Autodesk Inventor part; units mm, degrees
ref_plane "YZ Plane" through (0, 0, 0) normal (1, 0, 0) x (0, 1, 0)
ref_plane "XZ Plane" through (0, 0, 0) normal (0, 1, 0) x (-1, 0, 0)
ref_plane "XY Plane" through (0, 0, 0) normal (0, 0, 1) x (1, 0, 0)
sketch "Sketch1" plane through (0, 0, 0) normal (0, 1, 0) x (-1, 0, 0)
  line L0 (107.2514, 61.1758) -> (-112.4586, 61.1758)
  line L1 (-112.4586, 61.1758) -> (-112.4586, 42.1258)
  line L2 (-112.4586, 42.1258) -> (107.2514, 42.1258)
  line L3 (107.2514, 42.1258) -> (107.2514, 61.1758)
  point P0 (0, 0)
  dimension "d0" = 219.71
  dimension "d1" = 19.05
extrude "Extrusion1" add sketch "Sketch1" along normal blind 50.8
sketch "Sketch2" plane through (-107.2514, 0, 61.1758) normal (0, 0, 1) x (1, 0, 0)
  line L0 (0, 0) -> (219.71, 0)
  line L1 (0, 50.8) -> (219.71, 50.8)
  line L2 (0, 0) -> (0, 50.8)
  line L3 (219.71, 0) -> (219.71, 50.8)
  point P0 (107.2514, 0)
  point P1 (9.525, 38.1)
  point P2 (9.525, 12.7)
  point P3 (210.185, 12.7)
  point P4 (210.185, 38.1)
  dimension "d4" = 0
  dimension "d5" = 0
  dimension "d6" = 0
  dimension "d7" = 0
  dimension "d8" = 12.7
  dimension "d9" = 12.7
  dimension "d10" = 9.525
  dimension "d11" = 9.525
hole "Hole1" at (-97.7264, 38.1, 61.1758) at (-97.7264, 12.7, 61.1758) at (102.9336, 12.7, 61.1758) at (102.9336, 38.1, 61.1758) direction (0, 0, -1) diameter 6.35 end through all
sketch "Sketch3" plane through (-107.2514, 0, 61.1758) normal (0, 0, 1) x (1, 0, 0)
  line L0 (19.05, 44.45) -> (200.66, 44.45)
  line L1 (200.66, 44.45) -> (200.66, 6.35)
  line L2 (200.66, 6.35) -> (19.05, 6.35)
  line L3 (19.05, 6.35) -> (19.05, 44.45)
  line L4 (0, 0) -> (0, 50.8)
  line L5 (219.71, 0) -> (219.71, 50.8)
  line L6 (219.71, 50.8) -> (0, 50.8)
  line L7 (0, 0) -> (219.71, 0)
  point P0 (107.2514, 0)
  dimension "d19" = 19.05
  dimension "d20" = 19.05
  dimension "d21" = 6.35
  dimension "d22" = 6.35
extrude "Extrusion2" cut sketch "Sketch3" against normal blind 6.35 contours L0 L1 L2 L3
sketch "Sketch6" plane through (0, 50.8, 0) normal (0, 1, 0) x (1, 0, 0)
  line L0 (-88.2014, -54.8258) -> (-107.2514, -54.8258)
  line L1 (-107.2514, -54.8258) -> (-107.2514, -42.1258)
  line L2 (-107.2514, -42.1258) -> (-88.2014, -42.1258)
  line L3 (-88.2014, -42.1258) -> (-88.2014, -54.8258)
  line L4 (112.4586, -42.1258) -> (-107.2514, -42.1258)
  line L5 (-107.2514, -42.1258) -> (-107.2514, -61.1758)
  line L6 (112.4586, -54.8258) -> (93.4086, -54.8258)
  line L7 (93.4086, -54.8258) -> (93.4086, -42.1258)
  line L8 (93.4086, -42.1258) -> (112.4586, -42.1258)
  line L9 (112.4586, -42.1258) -> (112.4586, -54.8258)
  line L10 (112.4586, -61.1758) -> (112.4586, -42.1258)
  line L11 (-107.2514, -61.1758) -> (112.4586, -61.1758)
  point P0 (0, 0)
  dimension "d25" = 0
  dimension "d26" = 12.7
  dimension "d27" = 0
  dimension "d28" = 19.05
  dimension "d32" = 19.05
  dimension "d33" = 0
  dimension "d34" = 6.35
extrude "Extrusion3" cut sketch "Sketch6" against normal blind 76.2 contours L0 L1 L2 L3 | L4 L9 L6 L7
sketch "Sketch7" plane through (0, 0, 0) normal (0, -1, 0) x (1, 0, 0)
  line L0 (112.4586, 61.1758) -> (112.4586, 54.8258)
  line L1 (93.4086, 42.1258) -> (-88.2014, 42.1258)
  line L2 (-107.2514, 54.8258) -> (-107.2514, 61.1758)
  point P0 (0, 0)
  point P1 (61.6586, 51.6508)
  point P2 (-56.4514, 51.6508)
  dimension "d37" = 50.8
  dimension "d38" = 9.525
  dimension "d39" = 50.8
  dimension "d40" = 9.525
hole "Hole2" at (61.6586, 0, 51.6508) at (-56.4514, 0, 51.6508) direction (0, 1, 0) diameter 4.9149 depth 25.4 tip angle 118
sketch "Sketch8" plane through (0, 0, 0) normal (0, -1, 0) x (1, 0, 0)
  line L0 (112.4586, 61.1758) -> (112.4586, 54.8258)
  line L1 (93.4086, 42.1258) -> (-88.2014, 42.1258)
  point P0 (0, 0)
  point P1 (-1.8414, 51.6508)
  point P2 (-1.8414, 51.6508)
  dimension "d48" = 114.3
  dimension "d49" = 9.525
hole "Hole3" at (-1.8414, 0, 51.6508) direction (0, 1, 0) diameter 4.9149 depth 25.4 tip angle 118
properties part number "BottomWall"
Can you work these out from the model? Positions are in its coordinate system, mm. A direction names the side the tool comes from. Give positions to 0.01 mm unless a question says otherwise; leave off trailing zeros. Order: outer loops, then holes, each group sorted by start corner. A loop starts at its lowest first (then second) coordinate and runs counter-clockwise, first axis right, second up. Notation, with made-up numbers: (47.25, 87.5) - (53.25, 87.5) arc R10 ccw to (53.25, 106.5) - close; hole circle Ø1 at (56, -16). An arc over 180 degrees is marked (long way). Write each question's results on one line, items separated by ' | '.
1) On a 3-axis mill with a long thin cutter (end or side, diameter ignored), from which of +Z, -Z, +X, -X, +Y, -Y can I reach the whole of each face in a straight line? I mean faces 4 (the face through (-88.201, 25, 58)), 5 (the face through (-2.58, 12.878, 49.307)), 6 (the face through (-100.874, 13.113, 57.956)), 7 (the face through (-98, 26, 54.826)), 8 (the face through (93.409, 26, 49)). Say none if no direction works.
Final values:
face 4: +Z | face 5: -Y | face 6: +Z, -Z | face 7: -Z, -X, +Y, -Y | face 8: -Z, +X, +Y, -Y
2) Please list where these lines run through material, in increasing order: line 1 along X through (y, z) = (9, 52); line 2 along X through (y, z) = (38.1, 57.5); line 3 along Y through (x, z) = (-60.5, 60). Write a range as [from, to].
Final values:
line 1: x = [-88.2, -58.88], [-54.02, -4.27], [0.59, 59.23], [64.09, 93.41] | line 2: x = [-107.25, -100.9], [-94.55, -88.2], [93.41, 99.76], [106.11, 112.46] | line 3: y = [0, 6.35], [44.45, 50.8]
3) Suppose I cut it at C-C, the plane x = -66.5. Write out the boundary of the cut face in (y, z), then the cut area to 3 significant figures.
Final values:
outline: (0, 42.13) - (50.8, 42.13) - (50.8, 61.18) - (44.45, 61.18) - (44.45, 54.83) - (6.35, 54.83) - (6.35, 61.18) - (0, 61.18) - close | area: 726 mm^2
4) Suppose I cut it at D-D, the plane z = 59.25. Write out the boundary of the cut face in (x, y) (3 decimals), then the cut area to 3 significant figures.
Final values:
outline: (-107.251, 0) - (112.459, 0) - (112.459, 50.8) - (-107.251, 50.8) - close; hole circle Ø6.35 at (-97.726, 12.7); hole circle Ø6.35 at (-97.726, 38.1); hole (-88.201, 6.35) - (93.409, 6.35) - (93.409, 44.45) - (-88.201, 44.45) - close; hole circle Ø6.35 at (102.934, 12.7); hole circle Ø6.35 at (102.934, 38.1) | area: 4,120 mm^2
5) If we mould it in two halves opening along Y, with no side actions, what happens to faces 1 (the face through (-100.874, 38.513, 57.956)), 2 (the face through (4, 50.8, 52)), 3 (the face through (1, 48, 61.176))? For each: pulls with the +Y half, pulls with the -Y half, needs draft (parallel to the pull), parting line crosses it, or undercut.
Final values:
face 1: undercut | face 2: pulls with the +Y half | face 3: needs draft
6) I'm going to push flat-ended pins straight in: pin 1 Ø5.5 at (x, y) = (-97.73, 38.1) entering from +Z; pin 2 Ø8.5 at (x, y) = (102.93, 12.7) entering from -Z; pin 3 Ø6 at (x, y) = (-71, 19.5) entering from +Z; pin 4 Ø6.5 at (y, z) = (24, 46) entering from -X. Where does each tip first touch, or does it pass through?
Final values:
pin 1: passes through | pin 2: stops at z = 54.83 | pin 3: stops at z = 54.83 | pin 4: stops at x = -88.2
